from build123d import *

# Parameters (mm, degrees)
F0_R         = 5
F1_DEPTH     = 1
F2_DEPTH     = 2.5
F4_DEPTH     = 1.5
F5_T1_DEPTH  = 35.75
F5_T3_DEPTH  = 1
F5_T5_DEPTH  = 34.75
F5_T7_DEPTH  = 1
F5_T9_DEPTH  = 0.5
F5_S13_W     = 1.02
F5_S13_H     = 1.02
F5_T14_DEPTH = 1.02
F5_S19_W     = 1.02
F5_S19_H     = 1.02
F5_T20_DEPTH = 1.02
F5_T24_ANGLE = 180
F5_T26_ANGLE = 180
F5_T30_ANGLE = 180
F5_T35_DEPTH = 3.5
F5_T39_DEPTH = 38.25
F5_T46_DEPTH = 38.25
F5_T50_DEPTH = 3.5


# Not quite as in the source:
# - a fillet or chamfer that OpenCascade refuses, or shapes differently, is made with other operations: its cross-section is extruded or revolved along the edge and cut away or added


with BuildPart() as f1:
    # F0 (on Top) → F1 (new body)
    with BuildSketch(Plane.XY):
        with BuildLine():
            Line((-12.4595724046, -6.125), (23.2904275954, -6.125))
            ThreePointArc((23.2904275954, -6.125), (29.4154275954, 0), (23.2904275954, 6.125))
            Line((23.2904275954, 6.125), (-12.4595724046, 6.125))
            ThreePointArc((-12.4595724046, 6.125), (-18.5845724046, 0), (-12.4595724046, -6.125))
        make_face()
        with Locations((23.2904275954, 0)):
            Circle(F0_R, mode=Mode.SUBTRACT)
        with BuildLine():
            Line((-12.4595724046, -7.125), (-12.4595724046, -6.125))
            ThreePointArc((-12.4595724046, -6.125), (-18.5845724046, 0), (-12.4595724046, 6.125))
            Line((-12.4595724046, 6.125), (-12.4595724046, 7.125))
            ThreePointArc((-12.4595724046, 7.125), (-19.5845724046, 0), (-12.4595724046, -7.125))
        make_face()
    extrude(amount=F1_DEPTH)

    # F0 (on Top) → F2 (join)
    with BuildSketch(Plane.XY):
        with BuildLine():
            ThreePointArc((23.2904275954, 6.125), (29.4154275954, 0), (23.2904275954, -6.125))
            Line((23.2904275954, -6.125), (-12.4595724046, -6.125))
            Line((-12.4595724046, -6.125), (-12.4595724046, -7.125))
            Line((-12.4595724046, -7.125), (23.2904275954, -7.125))
            ThreePointArc((23.2904275954, -7.125), (30.4154275954, 0), (23.2904275954, 7.125))
            Line((23.2904275954, 7.125), (-12.4595724046, 7.125))
            Line((-12.4595724046, 7.125), (-12.4595724046, 6.125))
            Line((-12.4595724046, 6.125), (23.2904275954, 6.125))
        make_face()
    extrude(amount=F2_DEPTH)

    # F3 (on face) → F4 (join)
    with BuildSketch(Plane.XY.offset(2.5)):
        with BuildLine():
            Line((-12.4595724046, -7.125), (23.2904275954, -7.125))
            ThreePointArc((23.2904275954, -7.125), (30.4154275954, 0), (23.2904275954, 7.125))
            Line((23.2904275954, 7.125), (-12.4595724046, 7.125))
            Line((-12.4595724046, 7.125), (-12.4595724046, 6.125))
            Line((-12.4595724046, 6.125), (23.2904275954, 6.125))
            ThreePointArc((23.2904275954, 6.125), (29.4154275954, 0), (23.2904275954, -6.125))
            Line((23.2904275954, -6.125), (-12.4595724046, -6.125))
            Line((-12.4595724046, -6.125), (-12.4595724046, -7.125))
        make_face()
        with BuildLine():
            Line((-12.4595724046, -5.125), (-12.4595724046, -6.125))
            Line((-12.4595724046, -6.125), (23.2904275954, -6.125))
            ThreePointArc((23.2904275954, -6.125), (29.4154275954, 0), (23.2904275954, 6.125))
            Line((23.2904275954, 6.125), (-12.4595724046, 6.125))
            Line((-12.4595724046, 6.125), (-12.4595724046, 5.125))
            Line((-12.4595724046, 5.125), (23.2904275954, 5.125))
            ThreePointArc((23.2904275954, 5.125), (28.4154275954, 0), (23.2904275954, -5.125))
            Line((23.2904275954, -5.125), (-12.4595724046, -5.125))
        make_face()
    extrude(amount=F4_DEPTH)

    # F5: fillet of radius 1 on 12 edges, made by hand

    # F5_s2 → F5_t1 (cut)
    with BuildSketch(Plane.YZ.offset(-12.4595724046)):
        with BuildLine():
            ThreePointArc((-6.125, 4), (-6.8321067812, 3.7071067812), (-7.125, 3))
            Line((-7.125, 3), (-7.145, 3))
            Line((-7.145, 3), (-7.145, 4.02))
            Line((-7.145, 4.02), (-6.125, 4.02))
            Line((-6.125, 4.02), (-6.125, 4))
        make_face()
        with BuildLine():
            ThreePointArc((6.125, 4), (6.8321067812, 3.7071067812), (7.125, 3))
            Line((7.125, 3), (7.145, 3))
            Line((7.145, 3), (7.145, 4.02))
            Line((7.145, 4.02), (6.125, 4.02))
            Line((6.125, 4.02), (6.125, 4))
        make_face()
    extrude(amount=F5_T1_DEPTH, mode=Mode.SUBTRACT)

    # F5_s4 → F5_t3 (cut)
    with BuildSketch(Plane.XZ.offset(-7.125)):
        with BuildLine():
            ThreePointArc((-11.4595724046, 4), (-12.1666791858, 3.7071067812), (-12.4595724046, 3))
            Line((-12.4595724046, 3), (-12.4795724046, 3))
            Line((-12.4795724046, 3), (-12.4795724046, 4.02))
            Line((-12.4795724046, 4.02), (-11.4595724046, 4.02))
            Line((-11.4595724046, 4.02), (-11.4595724046, 4))
        make_face()
    extrude(amount=F5_T3_DEPTH, mode=Mode.SUBTRACT)

    # F5_s6 → F5_t5 (cut)
    with BuildSketch(Plane.YZ.offset(-11.4595724046)):
        with BuildLine():
            ThreePointArc((6.125, 4), (5.4178932188, 3.7071067812), (5.125, 3))
            Line((5.125, 3), (5.105, 3))
            Line((5.105, 3), (5.105, 4.02))
            Line((5.105, 4.02), (6.125, 4.02))
            Line((6.125, 4.02), (6.125, 4))
        make_face()
        with BuildLine():
            ThreePointArc((-6.125, 4), (-5.4178932188, 3.7071067812), (-5.125, 3))
            Line((-5.125, 3), (-5.105, 3))
            Line((-5.105, 3), (-5.105, 4.02))
            Line((-5.105, 4.02), (-6.125, 4.02))
            Line((-6.125, 4.02), (-6.125, 4))
        make_face()
    extrude(amount=F5_T5_DEPTH, mode=Mode.SUBTRACT)

    # F5_s8 → F5_t7 (cut)
    with BuildSketch(Plane.XZ.offset(6.125)):
        with BuildLine():
            ThreePointArc((-12.4595724046, 3), (-12.1666791858, 3.7071067812), (-11.4595724046, 4))
            Line((-11.4595724046, 4), (-11.4595724046, 4.02))
            Line((-11.4595724046, 4.02), (-12.4795724046, 4.02))
            Line((-12.4795724046, 4.02), (-12.4795724046, 3))
            Line((-12.4795724046, 3), (-12.4595724046, 3))
        make_face()
    extrude(amount=F5_T7_DEPTH, mode=Mode.SUBTRACT)

    # F5_s10 → F5_t9 (cut)
    with BuildSketch(Plane.XY.offset(2.5)):
        with BuildLine():
            ThreePointArc((-12.4595724046, -6.125), (-12.1666791858, -5.4178932188), (-11.4595724046, -5.125))
            Line((-11.4595724046, -5.125), (-11.4595724046, -5.105))
            Line((-11.4595724046, -5.105), (-12.4795724046, -5.105))
            Line((-12.4795724046, -5.105), (-12.4795724046, -6.125))
            Line((-12.4795724046, -6.125), (-12.4595724046, -6.125))
        make_face()
        with BuildLine():
            ThreePointArc((-11.4595724046, 5.125), (-12.1666791858, 5.4178932188), (-12.4595724046, 6.125))
            Line((-12.4595724046, 6.125), (-12.4795724046, 6.125))
            Line((-12.4795724046, 6.125), (-12.4795724046, 5.105))
            Line((-12.4795724046, 5.105), (-11.4595724046, 5.105))
            Line((-11.4595724046, 5.105), (-11.4595724046, 5.125))
        make_face()
    extrude(amount=F5_T9_DEPTH, mode=Mode.SUBTRACT)


with BuildPart() as f5_tool12:
    # F5_s13 → F5_t14 (new body)
    with BuildSketch(Plane.YZ.offset(-11.4595724046)):
        with Locations((5.615, 3.51)):
            Rectangle(F5_S13_W, F5_S13_H)
    extrude(amount=-F5_T14_DEPTH)

    # F5_s15 → F5_t16 (revolve, cut)
    with BuildSketch(Plane(origin=(-11.4595724046, 6.125, 3), x_dir=(0, 0.7071067812, -0.7071067812), z_dir=(0, 0.7071067812, 0.7071067812))):
        with BuildLine():
            ThreePointArc((0, -1), (1, 0), (0, 1))
            Line((0, 1), (0, -1))
        make_face()
    revolve(axis=Axis((-11.4595724046, 6.125, 3), (-1, 0, 0)), mode=Mode.SUBTRACT)


with BuildPart() as f1_1:
    add(f1.part)

    # F5_t11: cut F5_tool12
    add(f5_tool12.part, mode=Mode.SUBTRACT)


with BuildPart() as f5_tool18:
    # F5_s19 → F5_t20 (new body)
    with BuildSketch(Plane.XZ.offset(6.125)):
        with Locations((-11.9695724046, 3.51)):
            Rectangle(F5_S19_W, F5_S19_H)
    extrude(amount=-F5_T20_DEPTH)

    # F5_s21 → F5_t22 (revolve, cut)
    with BuildSketch(Plane(origin=(-11.4595724046, -6.125, 3), x_dir=(0.7071067812, 0, -0.7071067812), z_dir=(0.7071067812, 0, 0.7071067812))):
        with BuildLine():
            ThreePointArc((0, -1), (1, 0), (0, 1))
            Line((0, 1), (0, -1))
        make_face()
    revolve(axis=Axis((-11.4595724046, -6.125, 3), (0, 1, 0)), mode=Mode.SUBTRACT)


with BuildPart() as f1_2:
    add(f1_1.part)

    # F5_t17: cut F5_tool18
    add(f5_tool18.part, mode=Mode.SUBTRACT)

    # F5_s23 → F5_t24 (revolve, cut)
    with BuildSketch(Plane.YZ.offset(23.2904275954)):
        with BuildLine():
            ThreePointArc((-6.125, 4), (-6.8321067812, 3.7071067812), (-7.125, 3))
            Line((-7.125, 3), (-7.145, 3))
            Line((-7.145, 3), (-7.145, 4.02))
            Line((-7.145, 4.02), (-6.125, 4.02))
            Line((-6.125, 4.02), (-6.125, 4))
        make_face()
    revolve(axis=Axis((23.2904275954, 0, 4), (0, 0, 1)), revolution_arc=F5_T24_ANGLE, mode=Mode.SUBTRACT)

    # F5_s25 → F5_t26 (revolve, cut)
    with BuildSketch(Plane.YZ.offset(23.2904275954)):
        with BuildLine():
            ThreePointArc((6.125, 4), (5.4178932188, 3.7071067812), (5.125, 3))
            Line((5.125, 3), (5.105, 3))
            Line((5.105, 3), (5.105, 4.02))
            Line((5.105, 4.02), (6.125, 4.02))
            Line((6.125, 4.02), (6.125, 4))
        make_face()
    revolve(axis=Axis((23.2904275954, 0, 4), (0, 0, -1)), revolution_arc=F5_T26_ANGLE, mode=Mode.SUBTRACT)

    # F5_s27 → F5_t28 (revolve, cut)
    with BuildSketch(Plane.XZ):
        with BuildLine():
            ThreePointArc((29.2904275954, 1), (28.5833208142, 0.7071067812), (28.2904275954, 0))
            Line((28.2904275954, 0), (28.2704275954, 0))
            Line((28.2704275954, 0), (28.2704275954, 1.02))
            Line((28.2704275954, 1.02), (29.2904275954, 1.02))
            Line((29.2904275954, 1.02), (29.2904275954, 1))
        make_face()
    revolve(axis=Axis((23.2904275954, 0, 1), (0, 0, 1)), mode=Mode.SUBTRACT)

    # F5_s29 → F5_t30 (revolve, cut)
    with BuildSketch(Plane.YZ.offset(-12.4595724046)):
        with BuildLine():
            ThreePointArc((7.125, 0), (6.8321067812, 0.7071067812), (6.125, 1))
            Line((6.125, 1), (6.125, 1.02))
            Line((6.125, 1.02), (7.145, 1.02))
            Line((7.145, 1.02), (7.145, 0))
            Line((7.145, 0), (7.125, 0))
        make_face()
    revolve(axis=Axis((-12.4595724046, 0, 1), (0, 0, 1)), revolution_arc=F5_T30_ANGLE, mode=Mode.SUBTRACT)


with BuildPart() as f5_tool33:
    # F5_s34 → F5_t35 (new body)
    with BuildSketch(Plane.XZ.offset(6.125)):
        with BuildLine():
            ThreePointArc((-12.4595724046, 3), (-12.1666791858, 3.7071067812), (-11.4595724046, 4))
            Line((-11.4595724046, 4), (-11.4595724046, 4.02))
            Line((-11.4595724046, 4.02), (-12.4795724046, 4.02))
            Line((-12.4795724046, 4.02), (-12.4795724046, 3))
            Line((-12.4795724046, 3), (-12.4595724046, 3))
        make_face()
    extrude(amount=F5_T35_DEPTH)

    split(bisect_by=Plane.XZ.offset(7.125), keep=Keep.TOP)


with BuildPart() as f5_tool37:
    # F5_s38 → F5_t39 (new body)
    with BuildSketch(Plane.YZ.offset(-14.9595724046)):
        with BuildLine():
            ThreePointArc((-6.125, 4), (-6.8321067812, 3.7071067812), (-7.125, 3))
            Line((-7.125, 3), (-7.145, 3))
            Line((-7.145, 3), (-7.145, 4.02))
            Line((-7.145, 4.02), (-6.125, 4.02))
            Line((-6.125, 4.02), (-6.125, 4))
        make_face()
    extrude(amount=F5_T39_DEPTH)

    split(bisect_by=Plane.YZ.offset(-12.4595724046), keep=Keep.BOTTOM)


with BuildPart() as f5_tool33_1:
    add(f5_tool33.part)

    # F5_t41: intersect F5_tool37
    add(f5_tool37.part, mode=Mode.INTERSECT)


with BuildPart() as f1_3:
    add(f1_2.part)

    # F5_t31: cut F5_tool33
    add(f5_tool33_1.part, mode=Mode.SUBTRACT)


with BuildPart() as f5_tool44:
    # F5_s45 → F5_t46 (new body)
    with BuildSketch(Plane.YZ.offset(23.2904275954)):
        with BuildLine():
            ThreePointArc((6.125, 4), (6.8321067812, 3.7071067812), (7.125, 3))
            Line((7.125, 3), (7.145, 3))
            Line((7.145, 3), (7.145, 4.02))
            Line((7.145, 4.02), (6.125, 4.02))
            Line((6.125, 4.02), (6.125, 4))
        make_face()
    extrude(amount=-F5_T46_DEPTH)

    split(bisect_by=Plane.YZ.offset(-12.4595724046), keep=Keep.BOTTOM)


with BuildPart() as f5_tool48:
    # F5_s49 → F5_t50 (new body)
    with BuildSketch(Plane.XZ.offset(-9.625)):
        with BuildLine():
            ThreePointArc((-11.4595724046, 4), (-12.1666791858, 3.7071067812), (-12.4595724046, 3))
            Line((-12.4595724046, 3), (-12.4795724046, 3))
            Line((-12.4795724046, 3), (-12.4795724046, 4.02))
            Line((-12.4795724046, 4.02), (-11.4595724046, 4.02))
            Line((-11.4595724046, 4.02), (-11.4595724046, 4))
        make_face()
    extrude(amount=F5_T50_DEPTH)

    split(bisect_by=Plane.XZ.offset(-7.125), keep=Keep.BOTTOM)


with BuildPart() as f5_tool44_1:
    add(f5_tool44.part)

    # F5_t52: intersect F5_tool48
    add(f5_tool48.part, mode=Mode.INTERSECT)


with BuildPart() as f1_4:
    add(f1_3.part)

    # F5_t42: cut F5_tool44
    add(f5_tool44_1.part, mode=Mode.SUBTRACT)


solid = f1_4.part
Source: CAD feature listing. Evaluate the final solid. Frame: model axes, mm. A direction names the side the tool comes from. Give positions to 0.01 mm unless a question says otherwise; leave off trailing zeros. Write each loop counter-clockwise with the first axis right and the second up, starting at its lowest first coordinate (ties: lowest second). Pieces come first, ordered by that corner, then holes. Notation, with made-up numbers: M -23,56 L 22,56 A33 ccw 22,95 Z; hole C 84.25,63 d10. An arc over 180 degrees is marked long. Return JSON: item names as keys, results as strings. Group by question number.
1) Set-up query: faces 5 (the face through (30.414, -0.157, 1.479)), 6 (the face through (28.414, 0.113, 2.746)), 7 (the face through (29.414, 0.135, 1.74)). Return all of +Z, -Z, +X, -X, +Y, -Y with unobstructed straight access to the full face (end or side cutting, diameter ignored); none if empty.
2) Cut plane B-B, the plane z = 3.55. Output: boundary loops of the cut face in (x, y) (3 decimals), then the cut area to 3 significant figures.
3) Ray query, L1, parallel to Y at x = 15, z = 1.6 (3 decimals); L2, parallel to Y at x = 3, z = 2.8 (3 decimals); L3, parallel to Z at x = 22, y = 6. Return the intervals inside material, ascending.
4) Draft query along Y for faces 1 (the face through (-12.174, -5.426, 2.746)), 2 (the face through (-12.46, 6.6, 1.9)), 3 (the face through (5, -7.125, 1)), 4 (the face through (6, 7.125, 1)). Return one class per face: released by +Y, released by -Y, zero draft, split by the parting line, or undercut.
5) First-contact query: pin 1 Ø1 at (y, z) = (2.5, 2.5) entering from +X; pin 2 Ø1 at (x, y) = (-5, 3) entering from +Z. Flat tips, straight axial feed; report the tip coordinate or a pass-through.
6) Cut plane A-A, the plane x = 14.5. Output: boundary loops of the cut face in (y, z) (3 decimals), then the cut area to 3 significant figures.
Data:
{
 "1": {"face 5": "+Z, -Z, +X", "face 6": "+Z, -X", "face 7": "-X"},
 "2": {"outline": "M -12.295,-6.96 L 23.29,-6.96 A6.96 ccw 23.29,6.96 L -12.295,6.96 L -12.295,6.125 A0.835 ccw -11.46,5.29 L 23.29,5.29 A5.29 cw 23.29,-5.29 L -11.46,-5.29 A0.835 ccw -12.295,-6.125 Z", "area": "151 mm²"},
 "3": {"L1": "y = -7.125 to -6.125, 6.125 to 7.125", "L2": "y = -7.125 to -5.125, 5.125 to 7.125", "L3": "z = 0 to 1, 2.5 to 3.99"},
 "4": {"face 1": "undercut", "face 2": "zero draft", "face 3": "released by -Y", "face 4": "released by +Y"},
 "5": {"pin 1": "stops at x = 30.13", "pin 2": "stops at z = 1"},
 "6": {"outline": "M -7.125,0 L 7.125,0 L 7.125,3 A1 ccw 5.125,3 L 5.125,2.5 L 6.125,2.5 L 6.125,1 L -6.125,1 L -6.125,2.5 L -5.125,2.5 L -5.125,3 A1 ccw -7.125,3 Z", "area": "22.4 mm²"}
}
